from build123d import *

# Parameters (mm, degrees)
SKETCH1_W           = 155.702807198
SKETCH1_H           = 58
SKETCH1_R           = 1.5
BOSS_EXTRUDE2_DEPTH = 2
SKETCH2_W           = 5
SKETCH2_H           = 88
BOSS_EXTRUDE3_DEPTH = 2
SKETCH3_R           = 7.75
CUT_EXTRUDE1_DEPTH  = 10
SKETCH4_R           = 1.5
BOSS_EXTRUDE4_DEPTH = 2
SKETCH7_W           = 2.5
SKETCH7_H           = 88
CUT_EXTRUDE2_DEPTH  = 10


with BuildPart() as part:
    # Sketch1 → Boss-Extrude2 (new body)
    with BuildSketch(Plane(origin=(0, 0, 0), x_dir=(1, 0, 0), z_dir=(0, 1, 0))):
        with Locations((1.171695753, -5)):
            Rectangle(SKETCH1_W, SKETCH1_H)
        Polygon((-76.679707846, 44), (-76.679707846, 24), (79.023099352, 24), (79.023099352, 44), (62.885457038, 44), (59.885457038, 44), (-57.542065533, 44), (-60.542065533, 44), align=None)
        with Locations((-59.042065533, 34)):
            Circle(SKETCH1_R, mode=Mode.SUBTRACT)
        with Locations((61.385457038, 34)):
            Circle(SKETCH1_R, mode=Mode.SUBTRACT)
        Polygon((-76.679707846, -44), (-60.542065533, -44), (-57.542065533, -44), (59.885457038, -44), (62.885457038, -44), (79.023099352, -44), (79.023099352, -34), (-76.679707846, -34), align=None)
        with Locations((-59.042065533, -39)):
            Circle(SKETCH1_R, mode=Mode.SUBTRACT)
        with Locations((61.385457038, -39)):
            Circle(SKETCH1_R, mode=Mode.SUBTRACT)
    extrude(amount=BOSS_EXTRUDE2_DEPTH)

    # Sketch2 → Boss-Extrude3 (add)
    with BuildSketch(Plane(origin=(0, 2, 0), x_dir=(1, 0, 0), z_dir=(0, 1, 0))):
        with Locations((81.523099352, 0)):
            Rectangle(SKETCH2_W, SKETCH2_H)
        with Locations((-79.179707846, 0)):
            Rectangle(SKETCH2_W, SKETCH2_H)
    extrude(amount=-BOSS_EXTRUDE3_DEPTH)

    # Sketch3 → Cut-Extrude1 (cut)
    with BuildSketch(Plane(origin=(0, 2, 0), x_dir=(1, 0, 0), z_dir=(0, 1, 0))):
        with Locations((26.171695753, 13)):
            Circle(SKETCH3_R)
        with Locations((51.171695753, 13)):
            Circle(SKETCH3_R)
        with Locations((-23.828304247, 13)):
            Circle(SKETCH3_R)
        with Locations((-48.828304247, 13)):
            Circle(SKETCH3_R)
        with Locations((-48.828304247, -18)):
            Circle(SKETCH3_R)
        with Locations((-23.828304247, -18)):
            Circle(SKETCH3_R)
        with Locations((51.171695753, -18)):
            Circle(SKETCH3_R)
        with Locations((26.171695753, -18)):
            Circle(SKETCH3_R)
    extrude(amount=-CUT_EXTRUDE1_DEPTH, mode=Mode.SUBTRACT)

    # Sketch4 → Boss-Extrude4 (add)
    with BuildSketch(Plane(origin=(0, 2, 0), x_dir=(1, 0, 0), z_dir=(0, 1, 0))):
        Polygon((-23.828304247, 44), (26.171695753, 44), (26.171695753, 50.823606938), (13.671695753, 56.49492606), (-11.328304247, 56.49492606), (-23.828304247, 50.823606938), align=None)
        with Locations((1.171695753, 50.24746303)):
            Circle(SKETCH4_R, mode=Mode.SUBTRACT)
    extrude(amount=-BOSS_EXTRUDE4_DEPTH)

    # Sketch7 → Cut-Extrude2 (cut)
    with BuildSketch(Plane(origin=(0, 2, 0), x_dir=(1, 0, 0), z_dir=(0, 1, 0))):
        with Locations((-80.429707846, 0)):
            Rectangle(SKETCH7_W, SKETCH7_H)
        with Locations((82.773099352, 0)):
            Rectangle(SKETCH7_W, SKETCH7_H)
    extrude(amount=-CUT_EXTRUDE2_DEPTH, mode=Mode.SUBTRACT)


solid = part.part
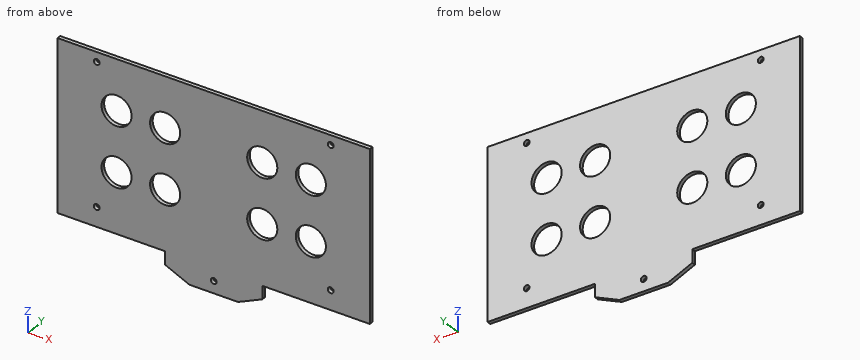
The model under review builds one solid part; all positions refer to its coordinate system, in mm. Coordinates: 2 decimals unless noted, no trailing zeros. Loops run counter-clockwise (first coordinate to the right, second up) from the corner with the lowest first, then second, coordinate; pieces in that order, holes last.
(1) Consider section A-A, the plane z = 18. Give the boundary of the cut face in (x, y), plus the area to 3 significant figures.
Determined:
outline: (-79.18, 0) - (-56.58, 0) - (-56.58, 2) - (-79.18, 2) - close; (-41.08, 0) - (-31.58, 0) - (-31.58, 2) - (-41.08, 2) - close; (-16.08, 0) - (18.42, 0) - (18.42, 2) - (-16.08, 2) - close; (33.92, 0) - (43.42, 0) - (43.42, 2) - (33.92, 2) - close; (58.92, 0) - (81.52, 0) - (81.52, 2) - (58.92, 2) - close
area: 197 mm2
(2) Consider section D-D, the plane z = -17.5. Give the boundary of the cut face in (x, y).
Determined:
outline: (-79.18, 0) - (-55.14, 0) - (-55.14, 2) - (-79.18, 2) - close; (-42.52, 0) - (-30.14, 0) - (-30.14, 2) - (-42.52, 2) - close; (-17.52, 0) - (19.86, 0) - (19.86, 2) - (-17.52, 2) - close; (32.48, 0) - (44.86, 0) - (44.86, 2) - (32.48, 2) - close; (57.48, 0) - (81.52, 0) - (81.52, 2) - (57.48, 2) - close
(3) Consider section C-C, the plane x = -63. Give the boundary of the cut face in (y, z).
Determined:
outline: (0, -44) - (2, -44) - (2, 44) - (0, 44) - close
(4) Insertion check: P1, Ø12.5, axis at x = -23.83, z = 18, coming from the +Y side; P2, Ø0.6, axis at x = -59, y = 1, coming from the -Z side; P3, Ø1, axis at y = 1.5, z = -47, coming from the -X side. Each pin has a flat end and moves straight along its axis. Give the tip position at first contact, or say it passes through.
Determined:
P1: passes through
P2: stops at z = -44
P3: stops at x = -23.83
(5) Consider section B-B, the plane y = 0.8. Give the number of separate pieces and of enclosed holes in the cut face, plus the area to 3 significant figures.
Determined:
separate pieces: 1
enclosed holes: 13
area: 13,200 mm2
(6) Wall thickness on L1, parallel to X at y = 0.9, z = 39; L2, parallel to X at y = 0.9, z = -16; L3, parallel to X at y = 0.5, z = -50.5: over which ranges is each line inside the solid? List them lowest first.
Determined:
L1: x = -79.18 to -60.54, -57.54 to 59.89, 62.89 to 81.52
L2: x = -79.18 to -55.97, -41.68 to -30.97, -16.68 to 19.03, 33.32 to 44.03, 58.32 to 81.52
L3: x = -23.83 to -0.31, 2.65 to 26.17
